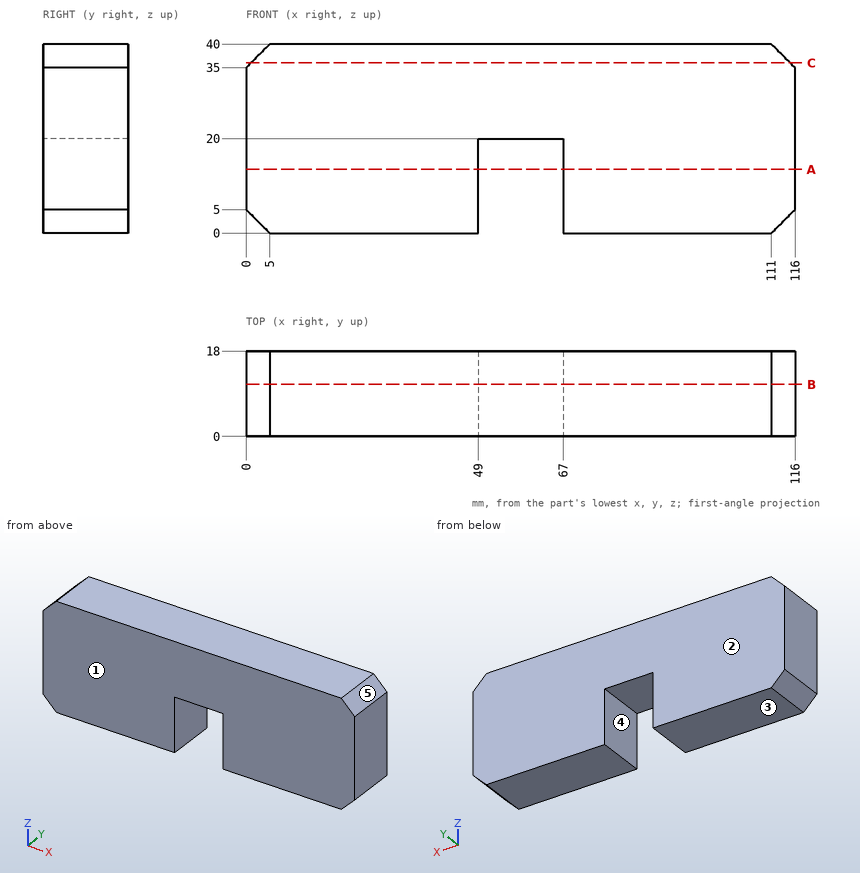
Can you work these out from the drawing? Everything is in mm from the part's minimum corner. A direction names the side the tool comes from. Round coordinates to 2 decimals unless told otherwise and drop trailing zeros. Loops run counter-clockwise (first coordinate to the right, second up) from the corner with the lowest first, then second, coordinate; pieces in that order, holes last. Notation, with made-up numbers: (17.5, 6) - (57.5, 6) arc R33 ccw to (57.5, 42) - close; hole circle Ø6 at (73, -0.75). An arc over 180 degrees is marked (long way). Write item = value, one per line. Start each with the question number.
(1) If I drill on probe 1 along X at (y, z) = (9.5, 9); probe 2 along Z at (x, y) = (62.5, 2.75); probe 3 along X at (y, z) = (9.25, 4.5), over which ranges is the centre line in solid material (lowest first)? Write a range as [from, to].
(2) If we section it at B-B (y = 11): Please give me the cut outline in (x, z), and give its area (3 significant figures).
(3) For the marked faces 4 and 5, which set-ups out of +Z, -Z, +X, -X, +Y, -Y let a thin tool reach every point of the face, with its end or its side?
(4) If we section it at C-C (z = 36): Please give me the cut outline in (x, y).
(5) If we mould it in two halves opening along Y, with no side actions, what happens to the marked faces 1, 2 and 3? For each: released by +Y, released by -Y, zero draft, split by the parting line, or undercut.
(6) If we section it at A-A (z = 13.5): Please give me the cut outline in (x, y).
Ans:
q1.probe_1 = [0, 49], [67, 116]
q1.probe_2 = [20, 40]
q1.probe_3 = [0.5, 49], [67, 115.5]
q2.outline = (0, 5) - (5, 0) - (49, 0) - (49, 20) - (67, 20) - (67, 0) - (111, 0) - (116, 5) - (116, 35) - (111, 40) - (5, 40) - (0, 35) - close
q2.area = 4,230 mm²
q3.face_4 = -Z, +Y, -Y
q3.face_5 = +Z, +X, +Y, -Y
q4.outline = (1, 0) - (115, 0) - (115, 18) - (1, 18) - close
q5.face_1 = released by -Y
q5.face_2 = released by +Y
q5.face_3 = zero draft
q6.outline = (0, 0) - (49, 0) - (49, 18) - (0, 18) - close; (67, 0) - (116, 0) - (116, 18) - (67, 18) - close
